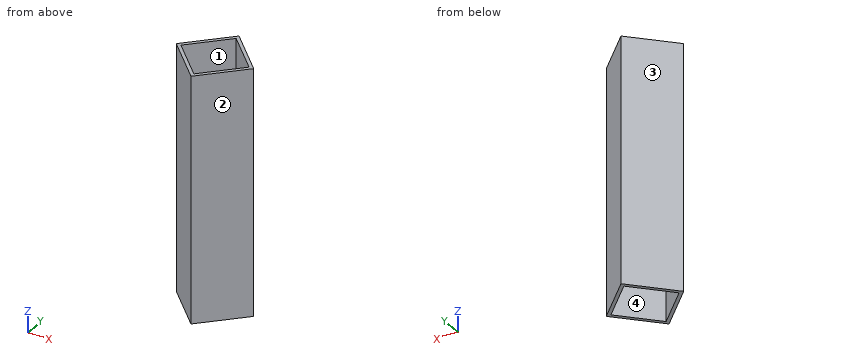
from build123d import *

# Parameters (mm, degrees)
EXTRUDE_1_DEPTH = 112.5


with BuildPart() as part:
    # 草圖1 → 填料-伸長1 (new body)
    with BuildSketch(Plane.XY):
        Polygon((0, 0), (17.69379362, -17.661530719), (0.032262901, -35.355324339), (-17.661530719, -17.69379362), align=None)
        Polygon((0.001935774, -2.12131946), (-15.540211259, -17.691857846), (0.030327127, -33.234004879), (15.57247416, -17.663466493), align=None, mode=Mode.SUBTRACT)
    extrude(amount=EXTRUDE_1_DEPTH)


solid = part.part
Could you check a few things on this model? Use its own coordinates, in mm. Face numbers are marked on the shaded views. Give positions to 0.01 mm unless a question says otherwise; leave off trailing zeros. Order: outer loops, then holes, each group sorted by start corner. A loop starts at its lowest first (then second) coordinate and runs counter-clockwise, first axis right, second up.
Item 1: I'm going to push flat-ended pins straight in: pin 1 (1.5 mm diameter, centred on x = -10.5, z = 55.5, fed in from -Y); pin 2 (10 mm diameter, centred on y = -25, z = 57, fed in from -X); pin 3 (5 mm diameter, centred on y = -20, z = 55.5, fed in from -X); pin 4 (6 mm diameter, centred on x = -9.5, z = 15, fed in from +Y). Where does each tip first touch, or does it pass through?
Item 2: If we mould it in two halves opening along Y, with no side actions, what happens to the marked faces 1, 2, 3 and 4? For each: pulls with the +Y half, pulls with the -Y half, needs draft (parallel to the pull), parting line crosses it, or undercut.
Item 3: If we section it at B-B, the plane y = -20.5: Write out the boundary of the cut face in (x, z), plus the area to 3 significant figures.
Item 4: I need wall thicknesses on line 1 (Y direction, x = -7, z = 59); line 2 (X direction, y = -23.5, z = 94); line 3 (X direction, y = -19, z = 40.5). Which ranges of each line are inside material? Lowest first, please.
Item 5: If we section it at C-C, the plane x = -3: Write out the boundary of the cut face in (y, z).
Item 6: If we section it at A-A, the plane z = 75.5: Write out the boundary of the cut face in (x, y).
Values:
1. pin 1: stops at y = -25.59
1. pin 2: stops at x = -15.35
1. pin 3: stops at x = -17.66
1. pin 4: stops at y = -6.51
2. face 1: undercut
2. face 2: pulls with the -Y half
2. face 3: pulls with the +Y half
2. face 4: undercut
3. outline: (-14.85, 0) - (-12.73, 0) - (-12.73, 112.5) - (-14.85, 112.5) - close; (12.74, 0) - (14.86, 0) - (14.86, 112.5) - (12.74, 112.5) - close
3. area: 477 mm2
4. line 1: y = -28.34 to -26.22, -9.14 to -7.01
4. line 2: x = -11.84 to -9.72, 9.75 to 11.87
4. line 3: x = -16.35 to -14.23, 14.24 to 16.36
5. outline: (-32.33, 0) - (-30.21, 0) - (-30.21, 112.5) - (-32.33, 112.5) - close; (-5.13, 0) - (-3.01, 0) - (-3.01, 112.5) - (-5.13, 112.5) - close
6. outline: (-17.66, -17.69) - (0.03, -35.36) - (17.69, -17.66) - (0, 0) - close; hole (-15.54, -17.69) - (0.03, -33.23) - (15.57, -17.66) - (0, -2.12) - close
